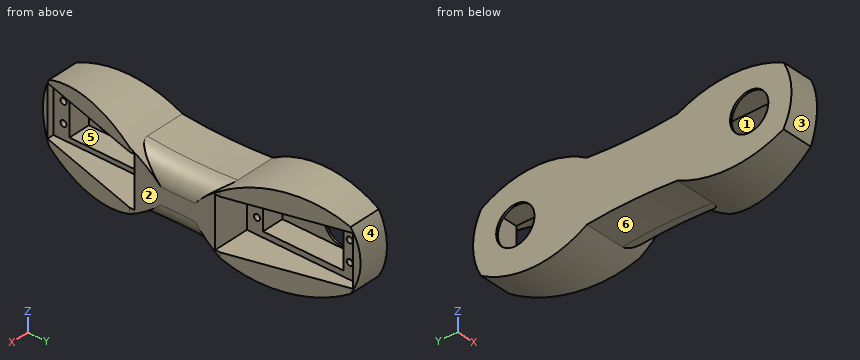
from build123d import *

# Parameters (mm, degrees)
BOSS_EXTRUDE1_DEPTH     = 30
SKETCH2_R               = 1.5000000000000049
SKETCH2_R_2             = 1.500000000000013
SKETCH2_R_3             = 1.5000000000000009
SKETCH2_R_4             = 1.5000000000000004
CUT_EXTRUDE1_DEPTH      = 29
CUT_EXTRUDE2_DEPTH      = 18
CUT_EXTRUDE3_DEPTH      = 40
CUT_EXTRUDE3_DEPTH_BACK = 40
SKETCH5_R               = 9.5
CUT_EXTRUDE4_DEPTH      = 40
FILLET1_R               = 10
FILLET2_R               = 10


with BuildPart() as part:
    # Sketch1 → Boss-Extrude1 (new body)
    with BuildSketch(Plane(origin=(0, 0, 0), x_dir=(0, 0, -1), z_dir=(1, 0, 0))):
        with BuildLine():
            ThreePointArc((14.999999999999988, 22.48862564156887), (13.986468943100135, -3.598e-14), (15, -22.488625641568866))
            ThreePointArc((15, -22.488625641568866), (21.049662737410323, -48.744312820784444), (15.000000000000004, -75.00000000000001))
            ThreePointArc((15.000000000000004, -75.00000000000001), (4.72e-15, -79.01923788646685), (-14.999999999999996, -75.00000000000001))
            ThreePointArc((-14.999999999999996, -75.00000000000001), (-21.049662737410294, -48.74431282078444), (-15.00000000000001, -22.488625641568866))
            ThreePointArc((-15.00000000000001, -22.488625641568866), (-13.986468943100135, 1.189e-14), (-15.00000000000001, 22.488625641568895))
            ThreePointArc((-15.00000000000001, 22.488625641568895), (-22.448397318700515, 48.74431282078445), (-15.000000000000007, 74.99999999999999))
            ThreePointArc((-15.000000000000007, 74.99999999999999), (-1.35e-15, 79.01923788646687), (14.99999999999999, 74.99999999999999))
            ThreePointArc((14.99999999999999, 74.99999999999999), (22.448397318700543, 48.744312820784415), (14.999999999999988, 22.48862564156887))
        make_face()
    extrude(amount=BOSS_EXTRUDE1_DEPTH)

    # Sketch2 → Cut-Extrude1 (cut)
    with BuildSketch(Plane(origin=(30, 0, 0), x_dir=(0, 0, -1), z_dir=(1, 0, 0))):
        with Locations((4.6684040574518, 71.01923788646675)):
            Circle(SKETCH2_R)
        with Locations((-5.331595942548199, 71.01923788646673)):
            Circle(SKETCH2_R_2)
        with Locations((4.6684040574518, 25.01923788646677)):
            Circle(SKETCH2_R_3)
        with Locations((-5.331595942548199, 24.86968442746252)):
            Circle(SKETCH2_R_4)
        with Locations((4.6684040574518, -25.019237886466854)):
            Circle(SKETCH2_R_3)
        with Locations((-5.331595942548199, -25.01923788646685)):
            Circle(SKETCH2_R_3)
        with Locations((4.6684040574518, -71.01923788646685)):
            Circle(SKETCH2_R_3)
        with Locations((-5.331595942548199, -71.01923788646685)):
            Circle(SKETCH2_R_3)
        Polygon((-10.3315959425482, 68.01923788646677), (9.6684040574518, 68.01923788646677), (9.668404057451806, 28.01923788646677), (-10.331595942548194, 28.019237886466765), align=None)
        Polygon((-10.331595942548196, -28.019237886466858), (9.668404057451804, -28.019237886466854), (9.66840405745181, -68.01923788646685), (-10.33159594254819, -68.01923788646685), align=None)
    extrude(amount=-CUT_EXTRUDE1_DEPTH, mode=Mode.SUBTRACT)

    # Sketch3 → Cut-Extrude2 (cut)
    with BuildSketch(Plane(origin=(30, 0, 0), x_dir=(0, 0, -1), z_dir=(1, 0, 0))):
        Polygon((-12.551602681299467, 76.01923788646684), (12.44839731870053, 76.01923788646684), (12.448397318700541, 20.019237886466833), (-12.55160268129946, 20.019237886466833), align=None)
        Polygon((-12.950337262589732, -20.01923788646686), (12.04966273741027, -20.01923788646686), (12.049662737410275, -76.01923788646687), (-12.950337262589725, -76.01923788646687), align=None)
    extrude(amount=-CUT_EXTRUDE2_DEPTH, mode=Mode.SUBTRACT)

    # Sketch4 → Cut-Extrude3 (cut, two sides: drawn at the far end of the back side and taken through both)
    with BuildSketch(Plane.XY.offset(-CUT_EXTRUDE3_DEPTH_BACK)):
        Polygon((15, 79.01923788646681), (30, 22.48862564156887), (30, -22.488625641568873), (14.279552603766648, -79.68148202341017), (43.09744845310124, -79.68148202341017), (43.09744845310124, 80.44995924605905), align=None)
    extrude(amount=CUT_EXTRUDE3_DEPTH + CUT_EXTRUDE3_DEPTH_BACK, mode=Mode.SUBTRACT)

    # Sketch5 → Cut-Extrude4 (cut)
    with BuildSketch(Plane(origin=(0, 0, 0), x_dir=(0, 0, -1), z_dir=(1, 0, 0))):
        with Locations((-0.33159594254819796, 58.01923788646677)):
            Circle(SKETCH5_R)
        with Locations((-0.331595942548191, -58.019237886466854)):
            Circle(SKETCH5_R)
    extrude(amount=CUT_EXTRUDE4_DEPTH, mode=Mode.SUBTRACT)

    # Fillet1
    # the kernel refuses this fillet: 10 mm, written as the material it takes off along each edge
    with BuildSketch(Plane(origin=(30, 7.017e-14, -263.9864689431014), x_dir=(0, 0.1889343030386976, 0.9819897296485751), z_dir=(0, 0.9819897296485751, -0.1889343030386976))) as fillet1_piece_1_section:
        with BuildLine():
            CenterArc((250.00000000000125 + FILLET1_R, -FILLET1_R), FILLET1_R, 90, 90)
            Line((250.00000000000125 + FILLET1_R, 0), (250.00000000000125, 0))
            Line((250.00000000000125, 0), (250.00000000000125, -FILLET1_R))
        make_face()
    fillet1_piece_1 = revolve(axis=Axis((30, 7.017e-14, -263.9864689431014), (1, 0, 0)), revolution_arc=21.781195760755132, mode=Mode.PRIVATE)
    fillet1_piece_1 = fillet1_piece_1 - Plane(origin=(27.494567227966037, 48.74431282078443, 27.551602681299116), x_dir=(0, 0.5251137435843147, -0.851032053625988), z_dir=(-1, 0, 0)) * Cylinder(49.99999999999966, 1041, mode=Mode.PRIVATE)
    fillet1_piece_1 = fillet1_piece_1 - Plane(origin=(27.494567227966037, -48.744312820784444, 38.95033726258946), x_dir=(0, 0.4375947863202612, -0.8991722877098276), z_dir=(-1, 0, 0)) * Cylinder(59.99999999999978, 1041, mode=Mode.PRIVATE)
    add(fillet1_piece_1, mode=Mode.SUBTRACT)

    # Fillet2
    fillet2_edges = [part.edges().sort_by_distance(p)[0] for p in [
        (30, 1.066e-14, 13.986468943100135),
    ]]
    fillet(fillet2_edges, radius=FILLET2_R)


solid = part.part
Geometry: final body of the model. Coordinates: model frame, mm. Face numbers are marked on the shaded views. A direction names the side the tool comes from. Give positions to 0.01 mm unless a question says otherwise; leave off trailing zeros. Loops run counter-clockwise (first coordinate to the right, second up) from the corner with the lowest first, then second, coordinate; pieces in that order, holes last. Notation, with made-up numbers: (57.5, 2) - (79.5, 2) arc R18 ccw to (79.5, 26) - close; hole circle Ø6 at (51.5, 26). An arc over 180 degrees is marked (long way). One line per question, with ' | ' between items. Start each with the question number.
(1) Section query D-D on y = 50.5. Return loops of the section in (x, z), then the cut area to 3 significant figures.
(2) Pull-direction query (Y, two-part tool) for the marked faces 1, 2, 3 and 4; classes: released by +Y, released by -Y, zero draft, split by the parting line, or undercut.
(3) Ray query, line 1 (Y direction, x = 14.5, z = -5.5); line 2 (Y direction, x = 14, z = -10); line 3 (X direction, y = -37, z = 8). Return the intervals inside material, ascending. Write a range as from..to.
(4) Section query B-B on y = -51. Return loops of the section in (x, z).
(5) Contact query for flat-ended pins moving along their axis: pin 1 (1.8 mm diameter, centred on y = -71.02, z = -4.67, fed in from -X); pin 2 (9 mm diameter, centred on x = 4, z = -4.5, fed in from -Y); pin 3 (16 mm diameter, centred on y = -43, z = 1, fed in from +X); pin 4 (6 mm diameter, centred on x = 21, z = 1.5, fed in from -Y). Output: stop coordinate, or through.
(6) Section query C-C on x = 5. Count the separate pieces of the cut face and the enclosed holes in it, then the cut area to 3 significant figures.
(7) Reachability of the marked faces 5 and 6 from +Z, -Z, +X, -X, +Y, -Y: full face, straight path, thin tool, end or side. Return the list, or none.
(8) Section query A-A on z = 17. Return loops of the section in (x, y), then the cut area to 3 significant figures.
The answers:
1) outline: (0, -22.42) - (22.57, -22.42) - (22.57, -12.45) - (12, -12.45) - (12, -9.67) - (1, -9.67) - (1, -5.47) - (0, -5.47) - close; (0, 6.14) - (1, 6.14) - (1, 10.33) - (12, 10.33) - (12, 12.55) - (22.57, 12.55) - (22.57, 22.42) - (0, 22.42) - close | area: 516 mm2
2) face 1: undercut | face 2: zero draft | face 3: released by -Y | face 4: released by +Y
3) line 1: -78.51..-76.02, -20.02..20.02, 76.02..78.51 | line 2: -77.3..-76.02, -20.02..20.02, 76.02..77.3 | line 3: 0..1
4) outline: (0, -21.01) - (22.16, -21.01) - (22.16, -12.05) - (12, -12.05) - (12, -9.67) - (1, -9.67) - (1, -6.07) - (0, -6.07) - close; (0, 6.73) - (1, 6.73) - (1, 10.33) - (12, 10.33) - (12, 12.95) - (22.16, 12.95) - (22.16, 21.01) - (0, 21.01) - close
5) pin 1: x = 0 | pin 2: y = -79.02 | pin 3: x = 1 | pin 4: y = -20.02
6) separate pieces: 1 | enclosed holes: 10 | area: 3,900 mm2
7) face 5: +X | face 6: -Z, +X, -X
8) outline: (0, -70.41) - (16.83, -70.41) - (28.74, -27.07) - (0, -27.07) - close; (0, 26.05) - (29.06, 26.05) - (17.01, 71.44) - (0, 71.44) - close | area: 2,030 mm2
